CAD build for the part. Positions are in the model's coordinates, mm. A direction names the side the tool comes from. Coordinates: 2 decimals unless noted, no trailing zeros. Order: outer loops, then holes, each group sorted by start corner. A loop starts at its lowest first (then second) coordinate and runs counter-clockwise, first axis right, second up. Notation, with made-up numbers: (28, -27) -> (35, -27) arc R33 cw to (35, 6) -> close; hole circle Ø7 at (53.25, 12.5). An arc over 180 degrees is marked (long way). Use one line per item in the form item = value. Start each with the question number.
from build123d import *

# Parameters (mm, degrees)
SKETCH1_W            = 300
SKETCH1_H            = 20
BOSS_EXTRUDE1_DEPTH  = 8
SKETCH2_W            = 34
SKETCH2_H            = 8
BOSS_EXTRUDE2_DEPTH  = 9
SKETCH3_W            = 34
SKETCH3_H            = 8
BOSS_EXTRUDE3_DEPTH  = 9
SKETCH4_R            = 1.5
CUT_EXTRUDE1_DEPTH   = 302.504560496
SKETCH5_W            = 25
SKETCH5_H            = 8
BOSS_EXTRUDE4_DEPTH  = 17
SKETCH6_W            = 25
SKETCH6_H            = 8
BOSS_EXTRUDE5_DEPTH  = 17
SKETCH7_W            = 10
SKETCH7_H            = 38
CUT_EXTRUDE2_DEPTH   = 303.37890138
SKETCH8_W            = 7
SKETCH8_H            = 16
CUT_EXTRUDE3_DEPTH   = 4
CUT_EXTRUDE4_DEPTH   = 7
BOSS_EXTRUDE6_DEPTH  = 10
SKETCH12_W           = 8
SKETCH12_H           = 8
BOSS_EXTRUDE7_DEPTH  = 17
SKETCH13_R           = 1.7
CUT_EXTRUDE6_DEPTH   = 305.926220585
SKETCH14_W           = 20
SKETCH14_H           = 12
BOSS_EXTRUDE8_DEPTH  = 12
SKETCH15_R           = 1.6
CUT_EXTRUDE7_DEPTH   = 20
SKETCH16_W           = 20
SKETCH16_H           = 12
BOSS_EXTRUDE9_DEPTH  = 12
SKETCH17_R           = 1.6
CUT_EXTRUDE8_DEPTH   = 20
SKETCH18_W           = 20
SKETCH18_H           = 13
BOSS_EXTRUDE10_DEPTH = 12
SKETCH19_R           = 1.6
CUT_EXTRUDE9_DEPTH   = 20
SKETCH20_W           = 20
SKETCH20_H           = 13
BOSS_EXTRUDE11_DEPTH = 12
SKETCH21_R           = 1.6
CUT_EXTRUDE10_DEPTH  = 20
FILLET6_R            = 3
SKETCH28_W           = 198.881436238
SKETCH28_H           = 556.355103816
CUT_EXTRUDE14_DEPTH  = 220
SKETCH29_W           = 21
SKETCH29_H           = 8
BOSS_EXTRUDE12_DEPTH = 15
SKETCH30_W           = 21
SKETCH30_H           = 10
CUT_EXTRUDE15_DEPTH  = 306.057371653
SKETCH31_R           = 1.6
CUT_EXTRUDE16_DEPTH  = 306.057371653
FILLET7_R            = 3
SKETCH32_W           = 5.5
SKETCH32_H           = 70.463459777
CUT_EXTRUDE17_DEPTH  = 0.8
SKETCH33_W           = 20
SKETCH33_H           = 4.963841857
CUT_EXTRUDE18_DEPTH  = 0.5
SKETCH34_W           = 20
SKETCH34_H           = 11.942443484
CUT_EXTRUDE19_DEPTH  = 0.5


with BuildPart() as part:
    # Sketch1 → Boss-Extrude1 (new body)
    with BuildSketch(Plane(origin=(0, 0, 0), x_dir=(1, 0, 0), z_dir=(0, 1, 0))):
        with Locations((150, -10)):
            Rectangle(SKETCH1_W, SKETCH1_H)
    extrude(amount=BOSS_EXTRUDE1_DEPTH)

    # Sketch2 → Boss-Extrude2 (add)
    with BuildSketch(Plane.XY.offset(20)):
        with Locations((17, 4)):
            Rectangle(SKETCH2_W, SKETCH2_H)
        with Locations((283, 4)):
            Rectangle(SKETCH2_W, SKETCH2_H)
    extrude(amount=BOSS_EXTRUDE2_DEPTH)

    # Sketch3 → Boss-Extrude3 (add)
    with BuildSketch(Plane(origin=(0, 0, 0), x_dir=(-1, 0, 0), z_dir=(0, 0, -1))):
        with Locations((-17, 4)):
            Rectangle(SKETCH3_W, SKETCH3_H)
        with Locations((-283, 4)):
            Rectangle(SKETCH3_W, SKETCH3_H)
    extrude(amount=BOSS_EXTRUDE3_DEPTH)

    # Sketch4 → Cut-Extrude1 (cut, through all)
    with BuildSketch(Plane(origin=(0, 8, 0), x_dir=(1, 0, 0), z_dir=(0, 1, 0))):
        with Locations(Location((4, 5, 0), (0, 0, 270))):
            Circle(SKETCH4_R)
        with Locations(Location((30, 5, 0), (0, 0, 270))):
            Circle(SKETCH4_R)
        with Locations(Location((30, -25, 0), (0, 0, 270))):
            Circle(SKETCH4_R)
        with Locations(Location((4, -25, 0), (0, 0, 270))):
            Circle(SKETCH4_R)
        with Locations(Location((296, -25, 0), (0, 0, 270))):
            Circle(SKETCH4_R)
        with Locations(Location((296, 5, 0), (0, 0, 270))):
            Circle(SKETCH4_R)
        with Locations(Location((270, -25, 0), (0, 0, 270))):
            Circle(SKETCH4_R)
        with Locations(Location((270, 5, 0), (0, 0, 270))):
            Circle(SKETCH4_R)
    extrude(amount=-CUT_EXTRUDE1_DEPTH, mode=Mode.SUBTRACT)

    # Sketch5 → Boss-Extrude4 (add)
    with BuildSketch(Plane.XY.offset(20)):
        with Locations((253.5, 4)):
            Rectangle(SKETCH5_W, SKETCH5_H)
    extrude(amount=BOSS_EXTRUDE4_DEPTH)

    # Sketch6 → Boss-Extrude5 (add)
    with BuildSketch(Plane(origin=(0, 0, 0), x_dir=(-1, 0, 0), z_dir=(0, 0, -1))):
        with Locations((-253.5, 4)):
            Rectangle(SKETCH6_W, SKETCH6_H)
    extrude(amount=BOSS_EXTRUDE5_DEPTH)

    # Sketch7 → Cut-Extrude2 (cut, through all)
    with BuildSketch(Plane(origin=(0, 8, 0), x_dir=(1, 0, 0), z_dir=(0, 1, 0))):
        with Locations((254, -10)):
            Rectangle(SKETCH7_W, SKETCH7_H)
    extrude(amount=-CUT_EXTRUDE2_DEPTH, mode=Mode.SUBTRACT)

    # Sketch8 → Cut-Extrude3 (cut)
    with BuildSketch(Plane(origin=(0, 8, 0), x_dir=(1, 0, 0), z_dir=(0, 1, 0))):
        with Locations((262.5, -10)):
            Rectangle(SKETCH8_W, SKETCH8_H)
    extrude(amount=-CUT_EXTRUDE3_DEPTH, mode=Mode.SUBTRACT)

    # Sketch9 → Cut-Extrude4 (cut)
    with BuildSketch(Plane.ZY.offset(-259)):
        Polygon((18, 4), (22, 8), (18, 8), align=None)
        Polygon((2, 4), (-2, 8), (2, 8), align=None)
    extrude(amount=-CUT_EXTRUDE4_DEPTH, mode=Mode.SUBTRACT)

    # Sketch10 → Boss-Extrude6 (add)
    with BuildSketch(Plane.ZY.offset(-259)):
        Polygon((-2, 0), (-9, 8), (-9, 0), align=None)
        Polygon((29, 8), (22, 0), (29, 0), align=None)
    extrude(amount=BOSS_EXTRUDE6_DEPTH)

    # Sketch12 → Boss-Extrude7 (add)
    with BuildSketch(Plane.XY.offset(37)):
        with Locations((245, 4)):
            Rectangle(SKETCH12_W, SKETCH12_H)
    extrude(amount=BOSS_EXTRUDE7_DEPTH)

    # Sketch13 → Cut-Extrude6 (cut, through all)
    with BuildSketch(Plane(origin=(0, 8, 0), x_dir=(1, 0, 0), z_dir=(0, 1, 0))):
        with Locations(Location((245, -50, 0), (0, 0, 270))):
            Circle(SKETCH13_R)
        with Locations(Location((245, -18, 0), (0, 0, 270))):
            Circle(SKETCH13_R)
    extrude(amount=-CUT_EXTRUDE6_DEPTH, mode=Mode.SUBTRACT)

    # Sketch14 → Boss-Extrude8 (add)
    with BuildSketch(Plane.XY.offset(29)):
        with Locations((285, 6)):
            Rectangle(SKETCH14_W, SKETCH14_H)
    extrude(amount=BOSS_EXTRUDE8_DEPTH)

    # Sketch15 → Cut-Extrude7 (cut)
    with BuildSketch(Plane(origin=(295, 0, 0), x_dir=(0, 0, -1), z_dir=(1, 0, 0))):
        with Locations((-35, 6)):
            Circle(SKETCH15_R)
    extrude(amount=-CUT_EXTRUDE7_DEPTH, mode=Mode.SUBTRACT)

    # Sketch16 → Boss-Extrude9 (add)
    with BuildSketch(Plane(origin=(0, 0, -9), x_dir=(-1, 0, 0), z_dir=(0, 0, -1))):
        with Locations((-285, 6)):
            Rectangle(SKETCH16_W, SKETCH16_H)
    extrude(amount=BOSS_EXTRUDE9_DEPTH)

    # Sketch17 → Cut-Extrude8 (cut)
    with BuildSketch(Plane(origin=(295, 0, 0), x_dir=(0, 0, -1), z_dir=(1, 0, 0))):
        with Locations((15, 6)):
            Circle(SKETCH17_R)
    extrude(amount=-CUT_EXTRUDE8_DEPTH, mode=Mode.SUBTRACT)

    # Sketch18 → Boss-Extrude10 (add)
    with BuildSketch(Plane(origin=(0, 0, -9), x_dir=(-1, 0, 0), z_dir=(0, 0, -1))):
        with Locations((-15, 6.5)):
            Rectangle(SKETCH18_W, SKETCH18_H)
    extrude(amount=BOSS_EXTRUDE10_DEPTH)

    # Sketch19 → Cut-Extrude9 (cut)
    with BuildSketch(Plane.ZY.offset(-5)):
        with Locations((-15, 8)):
            Circle(SKETCH19_R)
    extrude(amount=-CUT_EXTRUDE9_DEPTH, mode=Mode.SUBTRACT)

    # Sketch20 → Boss-Extrude11 (add)
    with BuildSketch(Plane.XY.offset(29)):
        with Locations((15, 6.5)):
            Rectangle(SKETCH20_W, SKETCH20_H)
    extrude(amount=BOSS_EXTRUDE11_DEPTH)

    # Sketch21 → Cut-Extrude10 (cut)
    with BuildSketch(Plane.ZY.offset(-5)):
        with Locations((35, 8)):
            Circle(SKETCH21_R)
    extrude(amount=-CUT_EXTRUDE10_DEPTH, mode=Mode.SUBTRACT)

    # Fillet6
    fillet6_edges = [part.edges().sort_by_distance(p)[0] for p in [
        (285, 12, 29),
        (285, 12, 41),
        (285, 12, -9),
        (285, 12, -21),
        (15, 13, -9),
        (15, 13, -21),
        (15, 13, 29),
        (15, 13, 41),
    ]]
    fillet(fillet6_edges, radius=FILLET6_R)

    # Sketch28 → Cut-Extrude14 (cut)
    with BuildSketch(Plane.ZY):
        with Locations((-20.495432896, -60.484201615)):
            Rectangle(SKETCH28_W, SKETCH28_H)
    extrude(amount=-CUT_EXTRUDE14_DEPTH, mode=Mode.SUBTRACT)

    # Sketch29 → Boss-Extrude12 (add)
    with BuildSketch(Plane(origin=(0, 0, 0), x_dir=(-1, 0, 0), z_dir=(0, 0, -1))):
        with Locations((-230.5, 4)):
            Rectangle(SKETCH29_W, SKETCH29_H)
    extrude(amount=BOSS_EXTRUDE12_DEPTH)

    # Sketch30 → Cut-Extrude15 (cut, through all)
    with BuildSketch(Plane(origin=(0, 0, 0), x_dir=(-1, 0, 0), z_dir=(0, -1, 0))):
        with Locations((-230.5, -15)):
            Rectangle(SKETCH30_W, SKETCH30_H)
    extrude(amount=-CUT_EXTRUDE15_DEPTH, mode=Mode.SUBTRACT)

    # Sketch31 → Cut-Extrude16 (cut, through all)
    with BuildSketch(Plane(origin=(0, 0, 0), x_dir=(-1, 0, 0), z_dir=(0, -1, 0))):
        with Locations(Location((-225, 7, 0), (0, 0, 90))):
            Circle(SKETCH31_R)
        with Locations(Location((-225, -3, 0), (0, 0, 90))):
            Circle(SKETCH31_R)
        with Locations(Location((-233, 7, 0), (0, 0, 90))):
            Circle(SKETCH31_R)
        with Locations(Location((-233, -3, 0), (0, 0, 90))):
            Circle(SKETCH31_R)
    extrude(amount=-CUT_EXTRUDE16_DEPTH, mode=Mode.SUBTRACT)

    # Fillet7
    fillet7_edges = [part.edges().sort_by_distance(p)[0] for p in [
        (300, 4, 29),
        (300, 4, -9),
    ]]
    fillet(fillet7_edges, radius=FILLET7_R)

    # Sketch32 → Cut-Extrude17 (cut)
    with BuildSketch(Plane(origin=(0, 12, 0), x_dir=(1, 0, 0), z_dir=(0, 1, 0))):
        with Locations((285, -7.2213573)):
            Rectangle(SKETCH32_W, SKETCH32_H)
    extrude(amount=-CUT_EXTRUDE17_DEPTH, mode=Mode.SUBTRACT)

    # Sketch33 → Cut-Extrude18 (cut)
    with BuildSketch(Plane(origin=(0, 0, 29), x_dir=(-1, 0, 0), z_dir=(0, 0, -1))):
        with Locations((-285, 10.481920928)):
            Rectangle(SKETCH33_W, SKETCH33_H)
    extrude(amount=-CUT_EXTRUDE18_DEPTH, mode=Mode.SUBTRACT)

    # Sketch34 → Cut-Extrude19 (cut)
    with BuildSketch(Plane.XY.offset(-9)):
        with Locations((285, 13.971221742)):
            Rectangle(SKETCH34_W, SKETCH34_H)
    extrude(amount=-CUT_EXTRUDE19_DEPTH, mode=Mode.SUBTRACT)


solid = part.part
1) Cut at A-A on z = 11. Give the cut face in (x, y), then the cut area to 3 significant figures.
2) Cut at B-B on x = 245. Give the cut face in (y, z), then the cut area to 3 significant figures.
3) 3-axis set-ups, long thin cutter, end or side, ignore diameter. For faces 5 (the face through (262, 6, 20)), 6 (the face through (296, 4, -9)), 7 (the face through (266, 4, -13)), 8 (the face through (285, 9, -9.5)): which of +Z, -Z, +X, -X, +Y, -Y reach the whole face in a straight line?
4) Two-plate mould, pull along X, no slides. Class faces 1 (the face through (249, 4, 45)), 2 (the face through (295, 4.6, -16.2)), 3 (the face through (226.08, 3.94, 4.18)), 4 (the face through (284.86, 10.69, -20.48)): released by +X, released by -X, zero draft, split by the parting line, or undercut.
5) Probe L1, parallel to Z at x = 225, y = 1.5; L2, parallel to Z at x = 270, y = 3; L3, parallel to X at y = 5, z = 25. List the from-to ranges inside material, lowest first.
6) Cut at C-C on z = 35. Give the cut face in (x, y).
7) Cut at D-D on z = 3. Give the cut face in (x, y), then the cut area to 3 significant figures.
8) Drop flat-ended pins along their axis: P1, Ø1, axis at x = 285.5, z = 0.5, coming from the +Y side; P2, Ø1.6, axis at x = 284, z = 36, coming from the +Y side; P3, Ø4, axis at y = 6, z = 44.5, coming from the +X side. Give the stop position or say it passes through.
Values follow:
q1.outline = (241, 0) -> (249, 0) -> (249, 8) -> (241, 8) -> close; (259, 0) -> (300, 0) -> (300, 8) -> (266, 8) -> (266, 4) -> (259, 4) -> close
q1.area = 364 mm^2
q2.outline = (0, -17) -> (8, -17) -> (8, 16.3) -> (0, 16.3) -> close; (0, 19.7) -> (8, 19.7) -> (8, 48.3) -> (0, 48.3) -> close; (0, 51.7) -> (8, 51.7) -> (8, 54) -> (0, 54) -> close
q2.area = 514 mm^2
q3.face_5 = +Y
q3.face_6 = -Z, +X, +Y, -Y
q3.face_7 = -Z, +Y, -Y
q3.face_8 = +X, -X, +Y
q4.face_1 = undercut
q4.face_2 = released by +X
q4.face_3 = undercut
q4.face_4 = zero draft
q5.L1 = -15 to -8.6, -5.4 to 1.4, 4.6 to 10
q5.L2 = -9 to -6.5, -3.5 to 23.5, 26.5 to 29
q5.L3 = 241 to 249, 259 to 268.5, 271.5 to 294.5, 297.5 to 300
q6.outline = (241, 0) -> (266, 0) -> (266, 8) -> (241, 8) -> close; (275, 0) -> (295, 0) -> (295, 4.4) -> (275, 4.4) -> close; (275, 7.6) -> (295, 7.6) -> (295, 12) -> (287.75, 12) -> (287.75, 11.2) -> (282.25, 11.2) -> (282.25, 12) -> (275, 12) -> close
q7.outline = (220, 0) -> (223.4, 0) -> (223.4, 8) -> (220, 8) -> close; (226.6, 0) -> (231.4, 0) -> (231.4, 8) -> (226.6, 8) -> close; (234.6, 0) -> (249, 0) -> (249, 8) -> (234.6, 8) -> close; (259, 0) -> (300, 0) -> (300, 8) -> (266, 8) -> (266, 4) -> (259, 4) -> close
q7.area = 481 mm^2
q8.P1 = 8
q8.P2 = 11.2
q8.P3 = 249
